Autodesk Inventor part; units mm, degrees
ref_plane "YZ Plane" through (0, 0, 0) normal (1, 0, 0) x (0, 1, 0)
ref_plane "XZ Plane" through (0, 0, 0) normal (0, 1, 0) x (-1, 0, 0)
ref_plane "XY Plane" through (0, 0, 0) normal (0, 0, 1) x (1, 0, 0)
sketch "Skizze1" plane through (0, 0, 0) normal (0, 0, 1) x (1, 0, 0)
  line L0 (0, 0) -> (-75, 0)
  line L1 (-75, 0) -> (-75, 16)
  line L2 (-75, 16) -> (0, 16)
  line L3 (0, 16) -> (0, 0)
  dimension "d0" = 75
  dimension "d1" = 16
extrude "Extrusion1" add sketch "Skizze1" along normal blind 5
sketch "Skizze2" plane through (0, 0, 5) normal (0, 0, 1) x (1, 0, 0)
  line L0 (0, 0) -> (0, 16) construction
  line L1 (-75, 0) -> (0, 0) construction
  line L2 (0, 0) -> (-75, 0) construction
  line L3 (-75, 0) -> (-75, 16) construction
  line L4 (-75, 16) -> (-75, 0) construction
  line L5 (-75, 16) -> (-59, 16) construction
  line L6 (-59, 16) -> (-59, 0) construction
  line L7 (-59, 16) -> (-75, 0) construction
  line L8 (-75, 16) -> (-59, 0) construction
  circle A0 centre (-67, 8) radius 8
  circle A1 centre (-67, 8) radius 6
  dimension "d4" = 16
  dimension "d5" = 16
  dimension "d6" = 16
  dimension "d7" = 12
extrude "Extrusion2" add sketch "Skizze2" along normal blind 30
sketch "Skizze3" plane through (-67, 8, 35) normal (0, 0, 1) x (1, 0, 0)
  circle A0 centre (0, 0) radius 6 construction
  line L0 (-6, 0) -> (6, 0) construction
  line L1 (0, 6) -> (0, -6) construction
  circle A1 centre (0, 0) radius 25
  circle A2 centre (0, 0) radius 6
  point P0 (67, -8)
  dimension "d10" = 50
extrude "Extrusion4" add sketch "Skizze3" along normal blind 5
sketch "Skizze4" plane through (0, 0, 5) normal (0, 0, 1) x (1, 0, 0)
  circle A0 centre (-67, 8) radius 6 construction
  line L0 (-67, 8) -> (-17, 8) construction
  line L1 (-17, 8) -> (-17, 13) construction
  line L2 (-17, 13) -> (-29, 13) construction
  line L3 (-29, 13) -> (-29, 3) construction
  line L4 (-29, 3) -> (-17, 3)
  line L5 (-17, 3) -> (-17, 13)
  line L6 (-17, 13) -> (-29, 13)
  line L7 (-29, 13) -> (-29, 3)
  point P0 (0, 0)
  dimension "d15" = 50
  dimension "d16" = 5
  dimension "d17" = 12
  dimension "d18" = 10
extrude "Extrusion5" add sketch "Skizze4" along normal blind 30
sketch "Skizze5" plane through (0, 0, 5) normal (0, 0, 1) x (1, 0, 0)
  circle A0 centre (-67, 8) radius 6 construction
  line L0 (-67, 8) -> (0, 8) construction
  line L1 (0, 0) -> (0, 16) construction
  line L2 (0, 8) -> (0, -29) construction
  line L3 (0, -29) -> (66, -29) construction
  line L4 (0, 8) -> (0, 28) construction
  line L5 (66, -29) -> (0, -29)
  line L6 (0, -29) -> (0, 28)
  line L7 (0, 28) -> (66, 28)
  line L8 (66, 28) -> (66, -29)
  dimension "d21" = 67
  dimension "d22" = 37
  dimension "d23" = 66
  dimension "d24" = 20
extrude "Extrusion6" add sketch "Skizze5" against normal blind 5
sketch "Skizze6" plane through (0, 0, 5) normal (0, 0, 1) x (1, 0, 0)
  line L0 (0, -29) -> (0, 0) construction
  line L1 (0, -29) -> (0, 15) construction
  line L2 (0, 15) -> (66, 15) construction
  line L3 (66, 28) -> (66, -29) construction
  line L4 (0, 15) -> (0, 5) construction
  line L5 (66, -29) -> (0, -29) construction
  line L6 (66, -29) -> (66, -19) construction
  line L7 (0, 5) -> (66, 5)
  line L8 (66, 5) -> (66, -19)
  line L9 (66, -19) -> (0, -19)
  line L10 (0, -19) -> (0, 5)
  dimension "d27" = 44
  dimension "d28" = 66
  dimension "d42" = 10
  dimension "d43" = 10
extrude "Extrusion7" add sketch "Skizze6" along normal blind 35
sketch "Skizze7" plane through (0, 0, 5) normal (0, 0, 1) x (1, 0, 0)
  line L0 (-67, 6.9194) -> (0, 7.5) construction
  line L1 (0, 0) -> (0, -19) construction
  line L2 (0, 7.5) -> (0, 22.5) construction
  line L3 (0, 22.5) -> (10, 22.5) construction
  line L4 (0, 28) -> (66, 28)
  line L5 (10, 22.5) -> (0, 22.5)
  line L6 (0, 22.5) -> (0, 28)
  line L7 (0, 28) -> (10, 28)
  line L8 (10, 28) -> (10, 22.5)
  point P0 (0, 15)
  dimension "d31" = 15
  dimension "d32" = 10
extrude "Extrusion8" add sketch "Skizze7" along normal blind 143
sketch "Skizze9" plane through (0, 0, 40) normal (0, 0, 1) x (1, 0, 0)
  line L0 (0, 0) -> (0, 5) construction
  line L1 (0, 5) -> (0, 15) construction
  line L2 (0, 15) -> (66, 15) construction
  line L3 (66, 28) -> (66, -29) construction
  line L4 (66, 15) -> (66, -29) construction
  line L5 (66, -29) -> (0, -29)
  line L6 (0, 15) -> (66, 15)
  line L7 (66, 15) -> (66, -29)
  line L8 (66, -29) -> (0, -29)
  line L9 (0, -29) -> (0, 15)
  dimension "d44" = 10
  dimension "d45" = 66
extrude "Extrusion10" add sketch "Skizze9" along normal blind 5
sketch "Skizze10" plane through (0, 0, 45) normal (0, 0, 1) x (1, 0, 0)
  circle A0 centre (-67, 8) radius 6 construction
  line L0 (-67, 8) -> (0, 8) construction
  line L1 (0, 8) -> (0, -7) construction
  line L2 (0, 0) -> (0, 5) construction
  line L3 (0, -7) -> (0, 13.3) construction
  line L4 (0, 13.3) -> (66, 13.3) construction
  line L5 (66, 28) -> (66, -29) construction
  line L6 (66, 13.3) -> (66, 6.8) construction
  line L7 (66, 6.8) -> (0, 6.8) construction
  line L8 (66, 5) -> (0, 5) construction
  line L9 (66, 6.8) -> (132, 6.8) construction
  line L10 (0, 13.3) -> (0, 6.8) construction
  line L11 (0, 5) -> (0, 15) construction
  line L12 (0, 13.3) -> (66, 13.3)
  line L13 (66, 13.3) -> (66, 6.8)
  line L14 (66, 6.8) -> (0, 6.8)
  line L15 (0, 6.8) -> (0, 13.3)
  dimension "d48" = 15
  dimension "d49" = 20.3
  dimension "d50" = 66
  dimension "d51" = 6.5
  dimension "d52" = 66
  dimension "d53" = 180
  dimension "d54" = 6.5
extrude "Extrusion11" add sketch "Skizze10" along normal blind 9
ref_plane "Arbeitsebene2" through (0, -7.9, 45) normal (0, -1, 0) x (1, 0, 0)
mirror "Spiegeln1" about plane through (0, -7.9, 45) normal (0, -1, 0) of "Extrusion11"
sketch "Skizze13" plane through (0, -29.1, 54) normal (0, 0, 1) x (1, 0, 0)
  circle A0 centre (14.0634, 3.7) radius 1.35
  circle A1 centre (36.0634, 3.7) radius 1.35
  circle A2 centre (58.0634, 3.7) radius 1.35
  circle A3 centre (14.0634, 3.7) radius 1.4
  circle A4 centre (36.0634, 3.7) radius 1.4
  circle A5 centre (58.0634, 3.7) radius 1.4
  point P0 (0, 29.1)
  dimension "d58" = 2.8
  dimension "d59" = 2.8
  dimension "d60" = 2.8
extrude "Extrusion12" cut sketch "Skizze13" against normal up to next contours A0 | A1 | A2 | A3 | A5
mirror "Spiegeln2" about plane through (0, -7.9, 45) normal (0, -1, 0) of "Extrusion12"
equation "\"d61\" = d60"
properties part number "base"
Geometry check sheet. Reference: the model listing, model coordinates, mm. A direction names the side the tool comes from. Round coordinates to 2 decimals unless told otherwise and drop trailing zeros. Order: outer loops, then holes, each group sorted by start corner. A loop starts at its lowest first (then second) coordinate and runs counter-clockwise, first axis right, second up. Notation, with made-up numbers: (-35.75, 10) - (17.25, 10) arc R18 ccw to (17.25, 19) - close; hole circle Ø3 at (26, 70.25). An arc over 180 degrees is marked (long way). Use a Markdown table: item, result. Add a question column.
1) Mould release check, pull along X, two halves, no side actions. Record for faces 1 (the flat face through (33, 15, 42)), 2 (the flat face through (-23, 3, 20)), 3 (the flat face through (10, 25, 75)): released by +X, released by -X, zero draft, split by the parting line, or undercut.
2) Thickness scan on line 1 along X through (y, z) = (9.6, 43.25); line 2 along Z through (x, y) = (6, 9); line 3 along Y through (x, z) = (54, 41.5). Record the ranges inside material, lowest first.
3) Section check D-D (x = 6). Record the cut outline in (y, z), then the cut area to 3 significant figures.
4) Section check A-A (z = 29). Record the cut outline in (x, y).
5) Section check C-C (y = 25.5). Record the cut outline in (x, z).
6) Set-up check for faces 4 (the flat face through (-29, 8, 20)), 5 (the flat face through (-73, 14, 35)), 6 (the cylindrical face through (-73, 8, 22)): record each of +Z, -Z, +X, -X, +Y, -Y from which the full face is reachable in a straight line by a thin tool's end or side.
7) Gauge pin test, flat ends, axial feed: P1, Ø2.5, axis at x = -72.5, y = 2, coming from the +Z side; P2, Ø7, axis at x = 24.5, y = -26, coming from the +Z side; P3, Ø1.5, axis at x = 47.5, z = 2.5, coming from the -Y side. Record the tip position at first contact, or that the pin passes through.
8) Section check B-B (x = -46). Record the cut outline in (y, z), then the cut area to 3 significant figures.
Established:
| question | item | result |
|---|---|---|
| 1 | face 1 | zero draft |
| 1 | face 2 | undercut |
| 1 | face 3 | released by +X |
| 2 | line 1 | 0 to 12.66, 15.46 to 34.71, 37.41 to 56.66, 59.46 to 66 |
| 2 | line 2 | 0 to 5, 40 to 54 |
| 2 | line 3 | -29 to 15 |
| 3 | outline | (-29.1, 45) - (-29, 45) - (-29, 40) - (-19, 40) - (-19, 5) - (-29, 5) - (-29, 0) - (28, 0) - (28, 148) - (22.5, 148) - (22.5, 5) - (5, 5) - (5, 40) - (15, 40) - (15, 45) - (13.3, 45) - (13.3, 54) - (6.8, 54) - (6.8, 45) - (-22.6, 45) - (-22.6, 54) - (-29.1, 54) - close |
| 3 | area | 2,250 mm2 |
| 4 | outline | circle Ø16 at (-67, 8); (-29, 3) - (-17, 3) - (-17, 13) - (-29, 13) - close; (0, -19) - (66, -19) - (66, 5) - (0, 5) - close; (0, 22.5) - (10, 22.5) - (10, 28) - (0, 28) - close; hole circle Ø12 at (-67, 8) |
| 5 | outline | (-84.85, 35) - (-49.15, 35) - (-49.15, 40) - (-84.85, 40) - close; (0, 0) - (66, 0) - (66, 5) - (10, 5) - (10, 148) - (0, 148) - close |
| 6 | face 4 | +Z, +Y, -Y |
| 6 | face 5 | none |
| 6 | face 6 | +Z |
| 7 | P1 | z = 40 |
| 7 | P2 | z = 54 |
| 7 | P3 | y = -29 |
| 8 | outline | (-5.56, 35) - (21.56, 35) - (21.56, 40) - (-5.56, 40) - close; (0, 0) - (16, 0) - (16, 5) - (0, 5) - close |
| 8 | area | 216 mm2 |
